Geometry check sheet. Reference: the model listing, model coordinates, mm. Give positions to 0.01 mm unless a question says otherwise; leave off trailing zeros. Write each loop counter-clockwise with the first axis right and the second up, starting at its lowest first coordinate (ties: lowest second). Pieces come first, ordered by that corner, then holes. Notation, with made-up numbers: M 41,83 L 91,83 A18 ccw 91,113 Z; hole C -3,56 d2. An arc over 180 degrees is marked long. Write each question's results on one line, items separated by ' | '.
```python
from build123d import *

# Parameters (mm, degrees)
SKETCH1_R           = 2.83
BOSS_EXTRUDE1_DEPTH = 2
CHAMFER1_SIZE       = 0.5
CHAMFER1_SIZE2      = 1.5


with BuildPart() as part:
    # Sketch1 → Boss-Extrude1 (new, symmetric)
    with BuildSketch(Plane.XY):
        Polygon((-81, -30), (50.07973639, -30), (50.07973639, 16.5), (57.3, 16.5), (57.3, 30), (-81, 30), align=None)
        with Locations((30, -24)):
            Circle(SKETCH1_R, mode=Mode.SUBTRACT)
    extrude(amount=BOSS_EXTRUDE1_DEPTH, both=True)

    # Chamfer1
    chamfer1_edges = [part.edges().sort_by_distance(p)[0] for p in [
        (27.17, -24, 2),
    ]]
    chamfer1_side = [part.faces().sort_by_distance(p)[0] for p in [
        (-14.755026682, 0.36160791, 2),
    ]]
    chamfer(chamfer1_edges, length=CHAMFER1_SIZE, length2=CHAMFER1_SIZE2, reference=chamfer1_side[0])


solid = part.part
```
Q1. Section check C-C (z = -0.15). Enter the section's corners in (x, y), then the cut area to 3 significant figures.
Answer key:
outline: M -81,-30 L 50.08,-30 L 50.08,16.5 L 57.3,16.5 L 57.3,30 L -81,30 Z; hole C 30,-24 d5.66 | area: 7,940 mm2
Q2. Depth check by flat-ended pin: P1, Ø1.2, axis at x = 52.5, z = 0.5, coming from the -Y side; P2, Ø2, axis at y = -7, z = 1, coming from the +X side. Enter the tip coordinate at first touch or a pass-through.
Answer key:
P1: stops at y = 16.5 | P2: stops at x = 50.08
Q3. Section check B-B (y = -24). Enter the section's corners in (x, z), then the cut area to 3 significant figures.
Answer key:
outline: M -81,-2 L 27.17,-2 L 27.17,0.5 L 26.67,2 L -81,2 Z; M 32.83,-2 L 50.08,-2 L 50.08,2 L 33.33,2 L 32.83,0.5 Z | area: 501 mm2
Q4. Release check for a two-part mould opening along X. For faces 1 (the face through (-81, 0, 0)), 2 (the face through (50.08, -7, 0)), 3 (the face through (28, -22, -1)), 4 (the face through (54, 16.5, 0)) record: released by +X, released by -X, zero draft, split by the parting line, or undercut.
Answer key:
face 1: released by -X | face 2: released by +X | face 3: undercut | face 4: zero draft
Q5. Section check A-A (x = 30). Enter the section's corners in (y, z), then the cut area to 3 significant figures.
Answer key:
outline: M -30,-2 L -26.83,-2 L -26.83,0.5 L -27.33,2 L -30,2 Z; M -21.17,-2 L 30,-2 L 30,2 L -20.67,2 L -21.17,0.5 Z | area: 217 mm2
Q6. Section check D-D (y = -18). Enter the section's corners in (x, z).
Answer key:
outline: M -81,-2 L 50.08,-2 L 50.08,2 L -81,2 Z
Q7. Material ranges on probe 1 along Y at (x, z) = (30, -1.4); probe 2 along X at (y, z) = (-26.5, -1.45); probe 3 along X at (y, z) = (-9, 0.35), recorded low to high. Write a range as [from, to].
Answer key:
probe 1: y = [-30, -26.83], [-21.17, 30] | probe 2: x = [-81, 28.67], [31.33, 50.08] | probe 3: x = [-81, 50.08]
